Could you check a few things on this drawing? It's one solid part, dimensions in mm from its lowest x, y, z. Give positions to 0.01 mm unless a question says otherwise; leave off trailing zeros. Order: outer loops, then holes, each group sorted by start corner. A loop starts at its lowest first (then second) coordinate and runs counter-clockwise, first axis right, second up.
Item 1: If I drill on line 1 along Y through (x, z) = (5, 18.2); line 2 along X through (y, z) = (30, 17.8); line 3 along Y through (x, z) = (67, 9), over which ranges is the centre line in solid material (lowest first)?
Item 2: I want a section at D-D, the plane x = 89. Write out the boundary of the cut face in (y, z), then the cut area to 3 significant figures.
Item 3: I want a section at A-A, the plane x = 115. Write out the boundary of the cut face in (y, z), then the cut area to 3 significant figures.
Item 4: I'm going to push flat-ended pins straight in: pin 1 Ø4 at (x, z) = (65.5, 15) entering from -Y; pin 2 Ø3 at (x, z) = (71, 16) entering from +Y; pin 3 Ø6.5 at (x, y) = (115, 5) entering from -Z; pin 4 Ø3.5 at (y, z) = (4, 16.5) entering from -X. Where does each tip first touch, or does it pass through?
Item 5: I want a section at B-B, the plane z = 12. Write out the boundary of the cut face in (x, y).
Item 6: I want a section at C-C, the plane y = 5. Write out the boundary of the cut face in (x, z).
Item 7: If we mould it in two halves opening along Y, with no side actions, what happens to the marked faces 1, 2 and 3? For each: +Y half, -Y half, draft (parallel to the pull), parting line (faces both ways), or undercut.
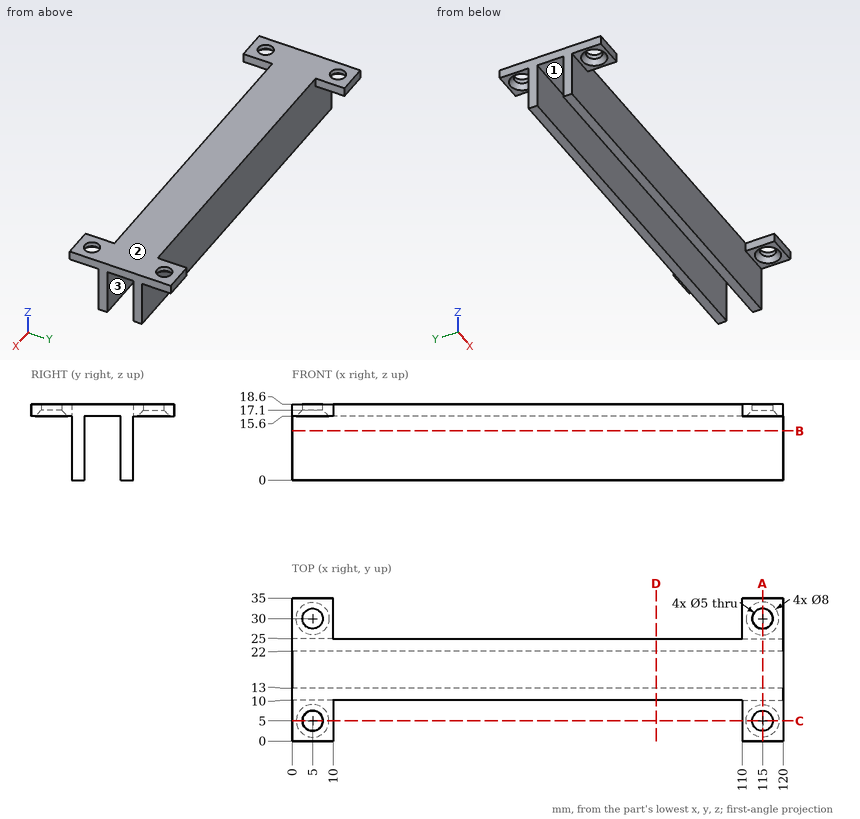
Results list:
1. line 1: y = 0 to 2.5, 7.5 to 27.5, 32.5 to 35
1. line 2: x = 0 to 2.5, 7.5 to 10, 110 to 112.5, 117.5 to 120
1. line 3: y = 10 to 13, 22 to 25
2. outline: (10, 0) - (13, 0) - (13, 15.6) - (22, 15.6) - (22, 0) - (25, 0) - (25, 18.6) - (10, 18.6) - close
2. area: 139 mm2
3. outline: (0, 15.6) - (1, 15.6) - (2.5, 17.1) - (2.5, 18.6) - (0, 18.6) - close; (7.5, 17.1) - (9, 15.6) - (10, 15.6) - (10, 0) - (13, 0) - (13, 15.6) - (22, 15.6) - (22, 0) - (25, 0) - (25, 15.6) - (26, 15.6) - (27.5, 17.1) - (27.5, 18.6) - (7.5, 18.6) - close; (32.5, 17.1) - (34, 15.6) - (35, 15.6) - (35, 18.6) - (32.5, 18.6) - close
3. area: 164 mm2
4. pin 1: stops at y = 10
4. pin 2: stops at y = 25
4. pin 3: stops at z = 16.35
4. pin 4: stops at x = 0
5. outline: (0, 10) - (120, 10) - (120, 13) - (0, 13) - close; (0, 22) - (120, 22) - (120, 25) - (0, 25) - close
6. outline: (0, 15.6) - (1, 15.6) - (2.5, 17.1) - (2.5, 18.6) - (0, 18.6) - close; (7.5, 17.1) - (9, 15.6) - (10, 15.6) - (10, 18.6) - (7.5, 18.6) - close; (110, 15.6) - (111, 15.6) - (112.5, 17.1) - (112.5, 18.6) - (110, 18.6) - close; (117.5, 17.1) - (119, 15.6) - (120, 15.6) - (120, 18.6) - (117.5, 18.6) - close
7. face 1: undercut
7. face 2: draft
7. face 3: undercut
